from build123d import *

# Parameters (mm, degrees)
SKETCH001_W   = 53
SKETCH001_H   = 44.5
PAD_DEPTH     = 2.88
SKETCH_W      = 6
SKETCH_H      = 18
SKETCH_W_2    = 10
PAD001_DEPTH  = 24.88
SKETCH002_W   = 53
SKETCH002_H   = 6.06
SKETCH003_W   = 32
SKETCH003_H   = 7.56
SKETCH003_W_2 = 15
SKETCH005_W   = 6
SKETCH005_H   = 6
SKETCH005_R   = 1.4
SKETCH005_W_2 = 10
SKETCH005_H_2 = 8.5
PAD002_DEPTH  = 24.88
SKETCH006_W   = 8.5
SKETCH006_H   = 4
PAD003_DEPTH  = 53
SKETCH007_R   = 1.4
POCKET_DEPTH  = 53.001


with BuildPart() as part:
    # Sketch001 → Pad (new body)
    with BuildSketch(Plane.XY):
        with Locations((26.5, -4.25)):
            Rectangle(SKETCH001_W, SKETCH001_H)
    extrude(amount=PAD_DEPTH)

    # Sketch → Pad001 (join)
    with BuildSketch(Plane.XY):
        with Locations((3, 9)):
            Rectangle(SKETCH_W, SKETCH_H)
        with Locations((35, 9)):
            Rectangle(SKETCH_W_2, SKETCH_H)
        with Locations((3, -17.5)):
            Rectangle(SKETCH_W, SKETCH_H)
        with Locations((18, -17.5)):
            Rectangle(SKETCH_W_2, SKETCH_H)
        with Locations((50, 9)):
            Rectangle(SKETCH_W, SKETCH_H)
        with Locations((50, -17.5)):
            Rectangle(SKETCH_W, SKETCH_H)
    extrude(amount=PAD001_DEPTH)

    # Sketch002 (on Face53 of Pad001) → Groove (revolve, cut)
    with BuildSketch(Plane.XY.offset(24.88)):
        with Locations((26.5, 12.03)):
            Rectangle(SKETCH002_W, SKETCH002_H)
    revolve(axis=Axis((0, 9, 24.88), (-1, 0, 0)), mode=Mode.SUBTRACT)

    # Sketch003 (on Face36 of Groove) → Groove001 (revolve, cut)
    with BuildSketch(Plane.XY.offset(24.88)):
        with Locations((18, 12.78)):
            Rectangle(SKETCH003_W, SKETCH003_H)
        with Locations((43.5, 12.78)):
            Rectangle(SKETCH003_W_2, SKETCH003_H)
    revolve(axis=Axis((0, 9, 24.88), (-1, 0, 0)), mode=Mode.SUBTRACT)

    # Sketch004 → Groove002 (revolve, cut)
    with BuildSketch(Plane.XY.offset(24.88)):
        Polygon((0, -17.5), (53, -17.5), (53, -11.44), (51, -11.44), (51, -9.94), (47, -9.94), (47, -11.44), (23, -11.44), (23, -9.94), (19, -9.94), (19, -11.44), (17, -11.44), (17, -9.94), (2, -9.94), (2, -11.44), (0, -11.44), align=None)
    revolve(axis=Axis((0, -17.5, 24.88), (1, 0, 0)), mode=Mode.SUBTRACT)

    # Sketch005 → Pad002 (join)
    with BuildSketch(Plane.XY):
        with Locations((3, -29.5)):
            Rectangle(SKETCH005_W, SKETCH005_H)
        with Locations((3, -29.5)):
            Circle(SKETCH005_R, mode=Mode.SUBTRACT)
        with Locations((18, -29.5)):
            Rectangle(SKETCH005_W_2, SKETCH005_H)
        with Locations((18, -29.5)):
            Circle(SKETCH005_R, mode=Mode.SUBTRACT)
        with Locations((50, -29.5)):
            Rectangle(SKETCH005_W, SKETCH005_H)
        with Locations((50, -29.5)):
            Circle(SKETCH005_R, mode=Mode.SUBTRACT)
        with Locations((3, 21)):
            Rectangle(SKETCH005_W, SKETCH005_H)
        with Locations((3, 21)):
            Circle(SKETCH005_R, mode=Mode.SUBTRACT)
        with Locations((35, 21)):
            Rectangle(SKETCH005_W_2, SKETCH005_H)
        with Locations((35, 21)):
            Circle(SKETCH005_R, mode=Mode.SUBTRACT)
        with Locations((50, 21)):
            Rectangle(SKETCH005_W, SKETCH005_H)
        with Locations((50, 21)):
            Circle(SKETCH005_R, mode=Mode.SUBTRACT)
        with Locations((3, -4.25)):
            Rectangle(SKETCH005_W, SKETCH005_H_2)
        with Locations((3, -4.25)):
            Circle(SKETCH005_R, mode=Mode.SUBTRACT)
        with Locations((18, -4.25)):
            Rectangle(SKETCH005_W_2, SKETCH005_H_2)
        with Locations((18, -4.25)):
            Circle(SKETCH005_R, mode=Mode.SUBTRACT)
        with Locations((35, -4.25)):
            Rectangle(SKETCH005_W_2, SKETCH005_H_2)
        with Locations((35, -4.25)):
            Circle(SKETCH005_R, mode=Mode.SUBTRACT)
        with Locations((50, -4.25)):
            Rectangle(SKETCH005_W, SKETCH005_H_2)
        with Locations((50, -4.25)):
            Circle(SKETCH005_R, mode=Mode.SUBTRACT)
    extrude(amount=PAD002_DEPTH)

    # Sketch006 → Pad003 (join)
    with BuildSketch(Plane.YZ):
        with Locations((-4.25, 2)):
            Rectangle(SKETCH006_W, SKETCH006_H)
    extrude(amount=PAD003_DEPTH)

    # Sketch007 → Pocket (cut, through all)
    with BuildSketch(Plane.YZ):
        with Locations((-2.125, 2)):
            Circle(SKETCH007_R)
        with Locations((-6.375, 2)):
            Circle(SKETCH007_R)
    extrude(amount=POCKET_DEPTH, mode=Mode.SUBTRACT)


solid = part.part
Part model, mm, in its own coordinate system. A direction names the side the tool comes from. Coordinates: 2 decimals unless noted, no trailing zeros. Loops run counter-clockwise (first coordinate to the right, second up) from the corner with the lowest first, then second, coordinate; pieces in that order, holes last. Notation, with made-up numbers: M -19.5,-17.5 L 37.5,-17.5 A5 cw 37.5,-10.5 Z; hole C -7.5,39 d7. An arc over 180 degrees is marked long. Use a Markdown table: item, result. Add a question column.
Q1. Pin check, flat tips, straight feed: P1, Ø6, axis at x = 39.5, y = 9.5, coming from the -Z side; P2, Ø2, axis at x = 43.5, y = -3.5, coming from the +Z side; P3, Ø2.5, axis at y = -14.5, z = 21.5, coming from the +X side; P4, Ø4, axis at x = 21.5, y = -16.5, coming from the +Z side. Stop position of each tip, or through.
Q2. Mould opens along Z. For faces 6 (the cylindrical face through (35.01, 9.13, 18.82)), 7 (the flat face through (40, 8, 12)), 8 (the cylindrical face through (26.129, -1.479, 0.758)) say: +Z half, -Z half, draft (parallel to the pull), parting line (faces both ways), or undercut.
Q3. Which spindle directions (+Z, -Z, +X, -X, +Y, -Y) get a long thin tool onto all of the face, cutting with end or side? Do faces 1 (the flat face through (2, -28, 24.88)), 2 (the flat face through (18, 0, 11)), 3 (the flat face through (35, -8.5, 11)), 4 (the flat face through (9, -26.5, 1)), 5 (the cylindrical face through (34.697, -5.617, 14.294)). Say none if no direction does.
Q4. Cut at C-C (z = 7). Give the number of separate pieces and of enclosed holes in the cut face, and give its area (3 significant figures).
Q5. Probe L1, parallel to X at y = 15, z = 17.75; L2, parallel to Y at x = 23.5, z = 2 (3 decimals); L3, parallel to Y at x = 50, z = 15.5. List the from-to ranges inside material, lowest first.
Q6. Cut at D-D (y = -29.5). Write the cut outline in (x, z), and give its area (3 significant figures).
Q7. Cut at B-B (x = 18). Write the cut outline in (y, z) (3 decimals).
Q8. Cut at A-A (x = 50). Write the cut outline in (y, z) (3 decimals), and give its area (3 significant figures).
Worked out:
| question | item | result |
|---|---|---|
| 1 | P1 | stops at z = 0 |
| 1 | P2 | stops at z = 4 |
| 1 | P3 | passes through |
| 1 | P4 | stops at z = 17.94 |
| 2 | face 6 | +Z half |
| 2 | face 7 | draft |
| 2 | face 8 | undercut |
| 3 | face 1 | +Z, +X, -X, +Y, -Y |
| 3 | face 2 | +Z, +Y |
| 3 | face 3 | +Z, -Y |
| 3 | face 4 | +Z, -Z, -Y |
| 3 | face 5 | +Z |
| 4 | separate pieces | 4 |
| 4 | enclosed holes | 10 |
| 4 | area | 1,270 mm2 |
| 5 | L1 | x = 0 to 6, 30 to 40, 47 to 53 |
| 5 | L2 | y = -26.5 to -7.775, -4.975 to -3.525, -0.725 to 18 |
| 5 | L3 | y = -32.5 to -30.9, -28.1 to -5.65, -2.85 to 19.6, 22.4 to 24 |
| 6 | outline | M 0,0 L 1.6,0 L 1.6,24.88 L 0,24.88 Z; M 4.4,0 L 6,0 L 6,24.88 L 4.4,24.88 Z; M 13,0 L 16.6,0 L 16.6,24.88 L 13,24.88 Z; M 19.4,0 L 23,0 L 23,24.88 L 19.4,24.88 Z; M 47,0 L 48.6,0 L 48.6,24.88 L 47,24.88 Z; M 51.4,0 L 53,0 L 53,24.88 L 51.4,24.88 Z |
| 6 | area | 338 mm2 |
| 7 | outline | M -32.5,0 L -30.9,0 L -30.9,24.88 L -32.5,24.88 Z; M -28.1,0 L 18,0 L 18,2.88 L 0,2.88 L 0,24.88 L -2.85,24.88 L -2.85,4 L -5.65,4 L -5.65,24.88 L -11.44,24.88 A6.06 cw -23.56,24.88 L -28.1,24.88 Z; hole C -6.375,2 d2.8; hole C -2.125,2 d2.8 |
| 8 | outline | M -32.5,0 L -30.9,0 L -30.9,24.88 L -32.5,24.88 Z; M -28.1,0 L 19.6,0 L 19.6,24.88 L 16.56,24.88 A7.56 cw 1.44,24.88 L -2.85,24.88 L -2.85,4 L -5.65,4 L -5.65,24.88 L -9.94,24.88 A7.56 cw -25.06,24.88 L -28.1,24.88 Z; M 22.4,0 L 24,0 L 24,24.88 L 22.4,24.88 Z; hole C -6.375,2 d2.8; hole C -2.125,2 d2.8 |
| 8 | area | 1,020 mm2 |
